CAD build for the part. Positions are in the model's coordinates, mm. A direction names the side the tool comes from. Give positions to 0.01 mm unless a question says otherwise; leave off trailing zeros. Order: outer loops, then holes, each group sorted by start corner. A loop starts at its lowest first (then second) coordinate and runs counter-clockwise, first axis right, second up.
```python
from build123d import *

# Parameters (mm, degrees)
BOSS_EXTRUDE1_DEPTH = 1
BOSS_EXTRUDE2_DEPTH = 1.6
SKETCH2_R           = 1.3
CUT_EXTRUDE1_DEPTH  = 2.6
SKETCH3_R           = 1.3
BOSS_EXTRUDE3_DEPTH = 1


with BuildPart() as part:
    # Sketch1 → Boss-Extrude1 (new body)
    with BuildSketch(Plane(origin=(0, 0, 0), x_dir=(1, 0, 0), z_dir=(0, 1, 0))):
        Polygon((-1.588897275, -2.752050808), (1.588897275, -2.752050808), (3.177794549, 0), (1.588897275, 2.752050808), (-1.588897275, 2.752050808), (-3.177794549, 0), align=None)
        Polygon((-1.30022214, -2.252050808), (1.30022214, -2.252050808), (2.60044428, 0), (1.30022214, 2.252050808), (-1.30022214, 2.252050808), (-2.60044428, 0), align=None, mode=Mode.SUBTRACT)
        Polygon((-2.60044428, 0), (-1.30022214, -2.252050808), (1.30022214, -2.252050808), (2.60044428, 0), (1.30022214, 2.252050808), (-1.30022214, 2.252050808), align=None)
        Polygon((-1, -1.732050808), (1, -1.732050808), (2, 0), (1, 1.732050808), (-1, 1.732050808), (-2, 0), align=None, mode=Mode.SUBTRACT)
        Polygon((-2, 0), (-1, -1.732050808), (1, -1.732050808), (2, 0), (1, 1.732050808), (-1, 1.732050808), align=None)
    extrude(amount=-BOSS_EXTRUDE1_DEPTH)

    # Sketch1_3 → Boss-Extrude2 (add)
    with BuildSketch(Plane(origin=(0, 0, 0), x_dir=(1, 0, 0), z_dir=(0, 1, 0))):
        Polygon((-1.588897275, -2.752050808), (1.588897275, -2.752050808), (3.177794549, 0), (1.588897275, 2.752050808), (-1.588897275, 2.752050808), (-3.177794549, 0), align=None)
        Polygon((-1.30022214, -2.252050808), (1.30022214, -2.252050808), (2.60044428, 0), (1.30022214, 2.252050808), (-1.30022214, 2.252050808), (-2.60044428, 0), align=None, mode=Mode.SUBTRACT)
    extrude(amount=BOSS_EXTRUDE2_DEPTH)

    # Sketch2 → Cut-Extrude1 (cut)
    with BuildSketch(Plane.XZ.offset(1)):
        with Locations(Location((0, 0, 0), (0, 0, 270))):
            Circle(SKETCH2_R)
    extrude(amount=-CUT_EXTRUDE1_DEPTH, mode=Mode.SUBTRACT)

    # Sketch3 → Boss-Extrude3 (add)
    with BuildSketch(Plane.XZ.offset(1)):
        Polygon((-1.588897275, -2.752050808), (1.588897275, -2.752050808), (3.177794549, 0), (1.588897275, 2.752050808), (-1.588897275, 2.752050808), (-3.177794549, 0), align=None)
        with Locations(Location((0, 0, 0), (0, 0, 270))):
            Circle(SKETCH3_R, mode=Mode.SUBTRACT)
    extrude(amount=BOSS_EXTRUDE3_DEPTH)


solid = part.part
```
Item 1: Slice it at D-D (x = 2). Give the cut face in (y, z), and give its area (3 significant figures).
Item 2: Drop flat-ended pins along their axis: pin 1 Ø1 at (y, z) = (-1, -1.5) entering from -X; pin 2 Ø1.6 at (x, z) = (0, 0) entering from +Y; pin 3 Ø1.5 at (y, z) = (0.5, -2) entering from +X. Give the stop position or say it passes through.
Item 3: Two-plate mould, pull along X, no slides. Class faces 3 (the face through (-1.94, 0.79, -1.14)), 4 (the face through (0, 0, 2.752)), 5 (the face through (-2.37, -0.17, 1.4)): released by +X, released by -X, zero draft, split by the parting line, or undercut.
Item 4: Slice it at B-B (y = 0.1). Give the cut face in (x, z), and give its area (3 significant figures).
Item 5: Slice it at C-C (z = 0.25). Give the cut face in (x, y), and give its area (3 significant figures).
Item 6: Wall check: L1, parallel to Z at x = 0.5, y = 1.15; L2, parallel to Y at x = -1.5, z = -1.85; L3, parallel to X at y = 1.4, z = 0.25. Give the ranges that are in metal, low to high.
Item 7: Tool access for faces 1 (the face through (2.394, -0.175, 1.357)), 2 (the face through (1.96, 0.79, -1.11)): list every direction of +Z, -Z, +X, -X, +Y, -Y with a clear straight run to the whole face (end or side of a thin tool).
Item 8: Slice it at A-A (x = 0). Give the cut face in (y, z).
A:
1. outline: (-2, -2.04) - (1.6, -2.04) - (1.6, -1.04) - (0, -1.04) - (0, 1.04) - (1.6, 1.04) - (1.6, 2.04) - (-2, 2.04) - close
1. area: 11.4 mm2
2. pin 1: stops at x = -2.6
2. pin 2: passes through
2. pin 3: stops at x = 2.46
3. face 3: undercut
3. face 4: zero draft
3. face 5: released by -X
4. outline: (-3.18, 0) - (-1.59, -2.75) - (1.59, -2.75) - (3.18, 0) - (1.59, 2.75) - (-1.59, 2.75) - close; hole (-2.6, 0) - (-1.3, -2.25) - (1.3, -2.25) - (2.6, 0) - (1.3, 2.25) - (-1.3, 2.25) - close
4. area: 8.67 mm2
5. outline: (-3.03, -2) - (-1.28, -2) - (-1.28, 0) - (-2.46, 0) - (-2.46, 1.6) - (-3.03, 1.6) - close; (1.28, -2) - (3.03, -2) - (3.03, 1.6) - (2.46, 1.6) - (2.46, 0) - (1.28, 0) - close
5. area: 8.88 mm2
6. L1: z = -2.75 to -2.25, 2.25 to 2.75
6. L2: y = -2 to 0
6. L3: x = -3.03 to -2.46, 2.46 to 3.03
7. face 1: +Z, +X, +Y, -Y
7. face 2: +Y
8. outline: (-2, -2.75) - (1.6, -2.75) - (1.6, -2.25) - (0, -2.25) - (0, -1.3) - (-2, -1.3) - close; (-2, 1.3) - (0, 1.3) - (0, 2.25) - (1.6, 2.25) - (1.6, 2.75) - (-2, 2.75) - close
